Can you work these out from the model? Positions are in its coordinate system, mm. Face numbers are marked on the shaded views. A direction names the side the tool comes from. Give positions to 0.01 mm unless a question says otherwise; leave off trailing zeros. Loops run counter-clockwise (first coordinate to the right, second up) from the corner with the lowest first, then second, coordinate; pieces in that order, holes last. Notation, with made-up numbers: M -35,51 L 3,51 A27 cw 3,67 Z; hole C 79.5,-38 d2. An arc over 180 degrees is marked long. Put each result on its own line as item: value. Start each with the question number.
1) Imagine slicing it at C-C (z = 4.5). Write out the boundary of the cut face in (x, y).
2) Imagine slicing it at D-D (x = -4.5). Write out the boundary of the cut face in (y, z), then the cut area to 3 significant figures.
3) Imagine slicing it at A-A (z = 0). Write out the boundary of the cut face in (x, y).
4) For P1, Ø0.7, axis at y = 7, z = 11, coming from the -X side; P2, Ø1.5, axis at y = 14.5, z = 4, coming from the -X side; P3, Ø1.2, axis at x = 1, y = 9, coming from the +Z side; P4, Ø4, axis at x = 2, z = 3, coming from the -Y side, each with a flat end and sliding along its axis, tell me the tip position at first contact or that it passes through.
5) Please list where these lines run through material, in increasing order: line 1 along Z through (x, y) = (0, 0.35); line 2 along Y through (x, z) = (-9, -6.25); line 3 along Z through (x, y) = (-11, 8). Write a range as from..to.
6) Imagine slicing it at B-B (x = 0). Write out the boundary of the cut face in (y, z).
7) For the marked faces 1, 2, 3, 4 and 5, which set-ups out of +Z, -Z, +X, -X, +Y, -Y let a thin tool reach every point of the face, with its end or its side?
from build123d import *

# Parameters (mm, degrees)
SKETCH1_R             = 12.55
BOSS_EXTRUDE1_DEPTH   = 1.5
SKETCH2_R             = 10.75
BOSS_EXTRUDE2_DEPTH   = 17.2
BOSS_EXTRUDE3_DEPTH   = 17.2
SKETCH4_R             = 3
BOSS_EXTRUDE4_DEPTH   = 1.61
SKETCH5_R             = 7
SKETCH5_R_2           = 6
CUT_EXTRUDE1_DEPTH    = 1
CHAMFER1_SIZE         = 7
CHAMFER1_SIZE2        = 1.234288865
CHAMFER1_PART_2_SIZE  = 7
CHAMFER1_PART_2_SIZE2 = 1.234288865
CHAMFER1_PART_3_SIZE  = 7
CHAMFER1_PART_3_SIZE2 = 1.234288865
CHAMFER1_PART_4_SIZE  = 7
CHAMFER1_PART_4_SIZE2 = 1.234288865


with BuildPart() as part:
    # Sketch1 → Boss-Extrude1 (new body)
    with BuildSketch(Plane(origin=(0, 0, 0), x_dir=(1, 0, 0), z_dir=(0, 1, 0))):
        Circle(SKETCH1_R)
    extrude(amount=BOSS_EXTRUDE1_DEPTH)

    # Sketch2 → Boss-Extrude2 (add)
    with BuildSketch(Plane(origin=(0, 1.5, 0), x_dir=(1, 0, 0), z_dir=(0, 1, 0))):
        Circle(SKETCH2_R)
    extrude(amount=BOSS_EXTRUDE2_DEPTH)

    # Sketch3 → Boss-Extrude3 (add)
    with BuildSketch(Plane(origin=(0, 1.5, 0), x_dir=(1, 0, 0), z_dir=(0, 1, 0))):
        with BuildLine():
            Line((2, 11.994879818), (-2, 11.994879818))
            Line((-2, 11.994879818), (-2, 10.562315087))
            ThreePointArc((-2, 10.562315087), (0, 10.75), (2, 10.562315087))
            Line((2, 10.562315087), (2, 11.994879818))
        make_face()
        with BuildLine():
            Line((-11.992315087, -2), (-11.992315087, 2))
            Line((-11.992315087, 2), (-10.562315087, 2))
            ThreePointArc((-10.562315087, 2), (-10.75, 0), (-10.562315087, -2))
            Line((-10.562315087, -2), (-11.992315087, -2))
        make_face()
        with BuildLine():
            Line((-2, -11.994879818), (-2, -10.562315087))
            ThreePointArc((-2, -10.562315087), (0, -10.75), (2, -10.562315087))
            Line((2, -10.562315087), (2, -11.994879818))
            Line((2, -11.994879818), (-2, -11.994879818))
        make_face()
        with BuildLine():
            Line((11.992315087, -2), (10.562315087, -2))
            ThreePointArc((10.562315087, -2), (10.75, 0), (10.562315087, 2))
            Line((10.562315087, 2), (11.992315087, 2))
            Line((11.992315087, 2), (11.992315087, -2))
        make_face()
    extrude(amount=BOSS_EXTRUDE3_DEPTH)

    # Sketch4 → Boss-Extrude4 (add)
    with BuildSketch(Plane(origin=(0, 18.7, 0), x_dir=(1, 0, 0), z_dir=(0, 1, 0))):
        with Locations((0, -4.5)):
            Circle(SKETCH4_R)
    extrude(amount=BOSS_EXTRUDE4_DEPTH)

    # Sketch5 → Cut-Extrude1 (cut)
    with BuildSketch(Plane.XZ):
        Circle(SKETCH5_R)
        Circle(SKETCH5_R_2, mode=Mode.SUBTRACT)
    extrude(amount=-CUT_EXTRUDE1_DEPTH, mode=Mode.SUBTRACT)

    # Chamfer1
    chamfer1_edges = [part.edges().sort_by_distance(p)[0] for p in [
        (0, 18.7, -11.994879818),
    ]]
    chamfer1_side = [part.faces().sort_by_distance(p)[0] for p in [
        (0, 10.1, -11.994879818),
    ]]
    chamfer(chamfer1_edges, length=CHAMFER1_SIZE, length2=CHAMFER1_SIZE2, reference=chamfer1_side[0])

    # Chamfer1 part 2
    chamfer1_part_2_edges = [part.edges().sort_by_distance(p)[0] for p in [
        (11.992315087, 18.7, 0),
    ]]
    chamfer1_part_2_side = [part.faces().sort_by_distance(p)[0] for p in [
        (11.992315087, 10.1, 0),
    ]]
    chamfer(chamfer1_part_2_edges, length=CHAMFER1_PART_2_SIZE, length2=CHAMFER1_PART_2_SIZE2, reference=chamfer1_part_2_side[0])

    # Chamfer1 part 3
    chamfer1_part_3_edges = [part.edges().sort_by_distance(p)[0] for p in [
        (-11.992315087, 18.7, 0),
    ]]
    chamfer1_part_3_side = [part.faces().sort_by_distance(p)[0] for p in [
        (-11.992315087, 10.1, 0),
    ]]
    chamfer(chamfer1_part_3_edges, length=CHAMFER1_PART_3_SIZE, length2=CHAMFER1_PART_3_SIZE2, reference=chamfer1_part_3_side[0])

    # Chamfer1 part 4
    chamfer1_part_4_edges = [part.edges().sort_by_distance(p)[0] for p in [
        (0, 18.7, 11.994879818),
    ]]
    chamfer1_part_4_side = [part.faces().sort_by_distance(p)[0] for p in [
        (0, 10.1, 11.994879818),
    ]]
    chamfer(chamfer1_part_4_edges, length=CHAMFER1_PART_4_SIZE, length2=CHAMFER1_PART_4_SIZE2, reference=chamfer1_part_4_side[0])


solid = part.part
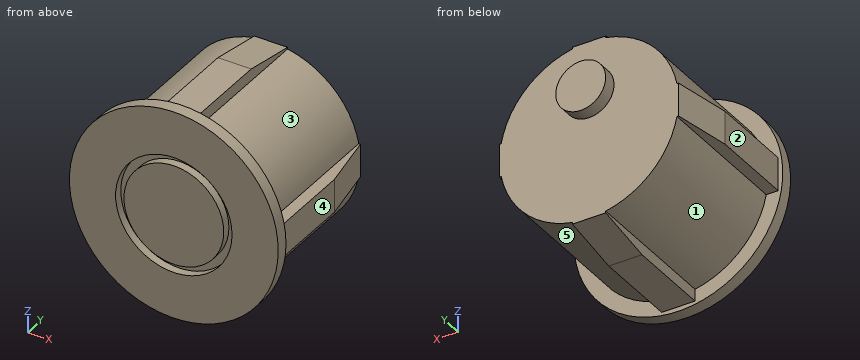
Recorded:
1. outline: M -11.72,0 L -5.36,0 L -5.36,1 L -3.97,1 L -3.97,0 L 3.97,0 L 3.97,1 L 5.36,1 L 5.36,0 L 11.72,0 L 11.72,1.5 L 9.76,1.5 L 9.76,18.7 L 3,18.7 L 3,20.31 L -3,20.31 L -3,18.7 L -9.76,18.7 L -9.76,1.5 L -11.72,1.5 Z
2. outline: M 0,-11.72 L 1.5,-11.72 L 1.5,-9.76 L 18.7,-9.76 L 18.7,9.76 L 1.5,9.76 L 1.5,11.72 L 0,11.72 L 0,5.36 L 1,5.36 L 1,3.97 L 0,3.97 L 0,-3.97 L 1,-3.97 L 1,-5.36 L 0,-5.36 Z
2. area: 368 mm²
3. outline: M -12.55,0 L -7,0 L -7,1 L -6,1 L -6,0 L 6,0 L 6,1 L 7,1 L 7,0 L 12.55,0 L 12.55,1.5 L 11.99,1.5 L 11.99,11.7 L 10.76,18.7 L -10.76,18.7 L -11.99,11.7 L -11.99,1.5 L -12.55,1.5 Z
4. P1: x = -2
4. P2: x = -10.25
4. P3: z = 11.99
4. P4: y = 0
5. line 1: -12.55..-7, -6..6, 7..12.55
5. line 2: 0..1.5
5. line 3: -2..2
6. outline: M 0,-12.55 L 1.5,-12.55 L 1.5,-11.99 L 11.7,-11.99 L 18.7,-10.76 L 18.7,1.5 L 20.31,1.5 L 20.31,7.5 L 18.7,7.5 L 18.7,10.76 L 11.7,11.99 L 1.5,11.99 L 1.5,12.55 L 0,12.55 L 0,7 L 1,7 L 1,6 L 0,6 L 0,-6 L 1,-6 L 1,-7 L 0,-7 Z
7. face 1: -Z, -X, +Y
7. face 2: +Z, -Z, -X, +Y
7. face 3: +Z, +X, +Y
7. face 4: +Z, -Z, +X, +Y
7. face 5: -Z, +X, +Y
